For this review, take the finished solid that the model builds, in its own axes (mm). A direction names the side the tool comes from. Coordinates: 2 decimals unless noted, no trailing zeros. Order: outer loops, then holes, each group sorted by start corner. A loop starts at its lowest first (then second) coordinate and runs counter-clockwise, first axis right, second up. Notation, with made-up numbers: (19.5, 22.25) - (26.5, 22.25) arc R14 ccw to (26.5, 49.25) - close; hole circle Ø5 at (61, -34.5). An arc over 180 degrees is marked (long way). One line per item, written item: value. Start each with the question number.
(1) To check wall thickness, follow line 1 along Z through (x, y) = (-0.05, -2); line 2 along X through (y, z) = (-7.25, 0.9); line 3 along X through (y, z) = (-4, -1.2). State the ranges of each line that lie inside material, in increasing order.
(2) Consider section A-A on y = -7. Write out the cut boundary in (x, z).
(3) Clearance check with flat-ended pins moving along their axes: pin 1 (3 mm diameter, centred on x = -1, y = -5, fed in from -Z); pin 2 (3 mm diameter, centred on y = -2, z = 0.5, fed in from -X); pin 3 (3 mm diameter, centred on y = -5, z = 2, fed in from +X). State where each tip first meets the part, or that it passes through.
(4) For faces 4 (the flat face through (0, -8, 0)), 5 (the flat face through (-0.605, -0.752, -0.008)), list the 3-axis set-ups (+Z, -Z, +X, -X, +Y, -Y) from which the entire face can be reached by the end or side of a thin tool; tool diameter is ignored.
(5) Mouldability with a two-part tool opening along Z and no side actions: class faces 1 (the flat face through (1.2, 0, 0)), 2 (the cylindrical face through (-0.45, -4.43, 1.43)), 3 (the flat face through (0.31, -0.75, -0.52)) as released by +Z, released by -Z, zero draft, split by the parting line, or undercut.
```python
from build123d import *
from OCP.BRepFilletAPI import BRepFilletAPI_MakeChamfer

# Parameters (mm, degrees)
SKETCH_4_R          = 1.5
EXTRUDE_2_DEPTH     = 8
CUT_EXTRUDE_1_DEPTH = 1.1
CHAMFER_3_SIZE      = 0.576368876
CHAMFER_3_SIZE2     = 0.998300177
CHAMFER_4_SIZE      = 0.3


with BuildPart() as part:
    # Sketch 2 → Revolve 1 (revolve)
    with BuildSketch(Plane.XY, mode=Mode.PRIVATE) as revolve_1_sk:
        Polygon((0, -1.86), (0, 0), (2.75, 0), (0.89, -1.86), align=None)
    revolve(revolve_1_sk.sketch.rotate(Axis((0, -1.86, 0), (0, 1, 0)), 270), axis=Axis((0, -1.86, 0), (0, 1, 0)))

    # Sketch 4 → Extrude 2 (add)
    with BuildSketch(Plane.XZ):
        with Locations(Location((0, 0, 0), (0, 0, 90))):
            Circle(SKETCH_4_R)
    extrude(amount=EXTRUDE_2_DEPTH)

    # Sketch 3 → Cut-Extrude 1 (cut)
    with BuildSketch(Plane(origin=(0, 0, 0), x_dir=(1, 0, 0), z_dir=(0, 1, 0))):
        Polygon((1, 0.577350269), (0, 1.154700538), (-1, 0.577350269), (-1, -0.577350269), (0, -1.154700538), (1, -0.577350269), align=None)
    extrude(amount=-CUT_EXTRUDE_1_DEPTH, mode=Mode.SUBTRACT)

    # Chamfer 3: one chamfer whose edges measure the first distance from different faces: ONE call of the kernel's chamfer builder (chamfer() names one face for all edges)
    chamfer_3_edges_1 = [part.edges().sort_by_distance(p)[0] for p in [
        (1, -1.1, 0),
    ]]
    chamfer_3_side_1 = [part.faces().sort_by_distance(p)[0] for p in [
        (1, -0.55, 0),
    ]]
    chamfer_3_edges_2 = [part.edges().sort_by_distance(p)[0] for p in [
        (0.5, -1.1, 0.866025404),
    ]]
    chamfer_3_side_2 = [part.faces().sort_by_distance(p)[0] for p in [
        (0.5, -0.55, 0.866025404),
    ]]
    chamfer_3_edges_3 = [part.edges().sort_by_distance(p)[0] for p in [
        (-0.5, -1.1, 0.866025404),
    ]]
    chamfer_3_side_3 = [part.faces().sort_by_distance(p)[0] for p in [
        (-0.5, -0.55, 0.866025404),
    ]]
    chamfer_3_edges_4 = [part.edges().sort_by_distance(p)[0] for p in [
        (-1, -1.1, 0),
    ]]
    chamfer_3_side_4 = [part.faces().sort_by_distance(p)[0] for p in [
        (-1, -0.55, 0),
    ]]
    chamfer_3_edges_5 = [part.edges().sort_by_distance(p)[0] for p in [
        (-0.5, -1.1, -0.866025404),
    ]]
    chamfer_3_side_5 = [part.faces().sort_by_distance(p)[0] for p in [
        (-0.5, -0.55, -0.866025404),
    ]]
    chamfer_3_edges_6 = [part.edges().sort_by_distance(p)[0] for p in [
        (0.5, -1.1, -0.866025404),
    ]]
    chamfer_3_side_6 = [part.faces().sort_by_distance(p)[0] for p in [
        (0.5, -0.55, -0.866025404),
    ]]
    chamfer_3 = BRepFilletAPI_MakeChamfer(part.part.solid().wrapped)
    for e in chamfer_3_edges_1:
        chamfer_3.Add(CHAMFER_3_SIZE, CHAMFER_3_SIZE2, e.wrapped, chamfer_3_side_1[0].wrapped)  # the first distance lies on this face
    for e in chamfer_3_edges_2:
        chamfer_3.Add(CHAMFER_3_SIZE, CHAMFER_3_SIZE2, e.wrapped, chamfer_3_side_2[0].wrapped)  # the first distance lies on this face
    for e in chamfer_3_edges_3:
        chamfer_3.Add(CHAMFER_3_SIZE, CHAMFER_3_SIZE2, e.wrapped, chamfer_3_side_3[0].wrapped)  # the first distance lies on this face
    for e in chamfer_3_edges_4:
        chamfer_3.Add(CHAMFER_3_SIZE, CHAMFER_3_SIZE2, e.wrapped, chamfer_3_side_4[0].wrapped)  # the first distance lies on this face
    for e in chamfer_3_edges_5:
        chamfer_3.Add(CHAMFER_3_SIZE, CHAMFER_3_SIZE2, e.wrapped, chamfer_3_side_5[0].wrapped)  # the first distance lies on this face
    for e in chamfer_3_edges_6:
        chamfer_3.Add(CHAMFER_3_SIZE, CHAMFER_3_SIZE2, e.wrapped, chamfer_3_side_6[0].wrapped)  # the first distance lies on this face
    add(Compound.cast(chamfer_3.Shape()), mode=Mode.REPLACE)

    # Chamfer 4
    chamfer_4_edges = [part.edges().sort_by_distance(p)[0] for p in [
        (0, -8, -1.5),
    ]]
    chamfer(chamfer_4_edges, length=CHAMFER_4_SIZE)


solid = part.part
```
Geometry check:
1. line 1: z = -1.5 to 1.5
1. line 2: x = -1.2 to 1.2
1. line 3: x = -0.9 to 0.9
2. outline: circle Ø3 at (0, 0)
3. pin 1: stops at z = -1.5
3. pin 2: stops at x = -2.22
3. pin 3: stops at x = 1.41
4. face 4: +Z, -Z, +X, -X, -Y
4. face 5: +Y
5. face 1: zero draft
5. face 2: split by the parting line
5. face 3: undercut
